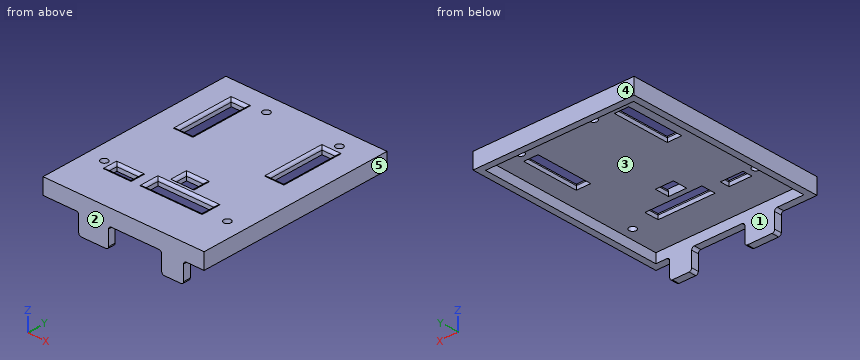
from build123d import *

# Parameters (mm, degrees)
SKETCH018_W   = 61.65
SKETCH018_H   = 75.98
SKETCH018_R   = 1.375
SKETCH018_W_2 = 21.82
SKETCH018_H_2 = 5.5
SKETCH018_W_3 = 8.7
SKETCH018_H_3 = 3.63
SKETCH018_W_4 = 6.9
SKETCH018_W_5 = 5.5
SKETCH018_H_4 = 21.975
SKETCH018_H_5 = 21.865
PAD011_DEPTH  = 2.5
SKETCH019_W   = 61.65
SKETCH019_H   = 75.98
SKETCH019_W_2 = 56.65
SKETCH019_H_2 = 70.73
PAD012_DEPTH  = 3.6
SKETCH020_W   = 11.43
SKETCH020_H   = 2.75
SKETCH020_W_2 = 8.39
PAD013_DEPTH  = 11.35
FILLET005_R   = 1


with BuildPart() as part:
    # Sketch018 → Pad011 (new body)
    with BuildSketch(Plane.XY):
        with Locations((0, -30.5)):
            Rectangle(SKETCH018_W, SKETCH018_H)
        with Locations((-8.89, 0.5)):
            Circle(SKETCH018_R, mode=Mode.SUBTRACT)
        with Locations((19.05, 0.5)):
            Circle(SKETCH018_R, mode=Mode.SUBTRACT)
        with Locations((-24.13, -50.3)):
            Circle(SKETCH018_R, mode=Mode.SUBTRACT)
        with Locations((24.13, -51.57)):
            Circle(SKETCH018_R, mode=Mode.SUBTRACT)
        with Locations((4.49, -49.92)):
            Rectangle(SKETCH018_W_2, SKETCH018_H_2, mode=Mode.SUBTRACT)
        with Locations((-16.12, -50.855)):
            Rectangle(SKETCH018_W_3, SKETCH018_H_3, mode=Mode.SUBTRACT)
        with Locations((1.03, -42.42)):
            Rectangle(SKETCH018_W_4, SKETCH018_H_2, mode=Mode.SUBTRACT)
        with Locations((-18.4, -11.7825)):
            Rectangle(SKETCH018_W_5, SKETCH018_H_4, mode=Mode.SUBTRACT)
        with Locations((18.475, -14.0775)):
            Rectangle(SKETCH018_W_5, SKETCH018_H_5, mode=Mode.SUBTRACT)
    extrude(amount=PAD011_DEPTH)

    # Sketch019 → Pad012 (join)
    with BuildSketch(Plane.XY):
        with Locations((0, -30.5)):
            Rectangle(SKETCH019_W, SKETCH019_H)
        with Locations((0, -30.375)):
            Rectangle(SKETCH019_W_2, SKETCH019_H_2, mode=Mode.SUBTRACT)
    extrude(amount=-PAD012_DEPTH)

    # Sketch020 → Pad013 (join)
    with BuildSketch(Plane.XY):
        with Locations((-11.43, -67.115)):
            Rectangle(SKETCH020_W, SKETCH020_H)
        with Locations((18.8, -67.115)):
            Rectangle(SKETCH020_W_2, SKETCH020_H)
    extrude(amount=-PAD013_DEPTH)

    # Fillet005
    fillet005_edges = [part.edges().sort_by_distance(p)[0] for p in [
        (-20.47, -50.855, 2.5),
        (-16.12, -49.04, 2.5),
        (-16.12, -52.67, 2.5),
        (-11.77, -50.855, 2.5),
        (-6.42, -49.92, 2.5),
        (4.49, -47.17, 2.5),
        (4.49, -52.67, 2.5),
        (15.4, -49.92, 2.5),
        (-2.42, -42.42, 2.5),
        (1.03, -39.67, 2.5),
        (4.48, -42.42, 2.5),
        (18.475, -3.145, 2.5),
        (21.225, -14.0775, 2.5),
        (15.725, -14.0775, 2.5),
        (18.475, -25.01, 2.5),
        (-18.4, -0.795, 2.5),
        (-15.65, -11.7825, 2.5),
        (-21.15, -11.7825, 2.5),
        (-18.4, -22.77, 2.5),
        (-17.145, -67.115, -3.6),
        (-17.145, -67.115, -11.35),
        (-5.715, -67.115, -11.35),
        (14.605, -67.115, -3.6),
        (14.605, -67.115, -11.35),
        (22.995, -67.115, -11.35),
        (-5.715, -67.115, -3.6),
        (22.995, -67.115, -3.6),
    ]]
    fillet(fillet005_edges, radius=FILLET005_R)


solid = part.part
The model under review builds one solid part; all positions refer to its coordinate system, in mm. Face numbers are marked on the shaded views. A direction names the side the tool comes from. Round coordinates to 2 decimals unless told otherwise and drop trailing zeros. Write each loop counter-clockwise with the first axis right and the second up, starting at its lowest first coordinate (ties: lowest second). Pieces come first, ordered by that corner, then holes. Notation, with made-up numbers: (-14.5, 49.25) - (11.5, 49.25) arc R15 ccw to (11.5, 64.25) - close; hole circle Ø7 at (-38.5, 26). An arc over 180 degrees is marked (long way). One line per item, written item: value. Start each with the question number.
1. Consider section C-C on z = -8.5. Write out the cut boundary in (x, y) (3 decimals).
2. Machinability: for the marked faces 1 and 2, which of the approach directions +Z, -Z, +X, -X, +Y, -Y give a long, thin tool a straight path to every point of the face, cutting with its end or side? Answer none if there is none.
3. The part is to be moulded in two halves that separate along X. For the marked faces 3, 4 and 5, say which applies: released by +X, released by -X, zero draft, split by the parting line, or undercut.
4. Consider section B-B on z = -1.75. Write out the cut boundary in (x, y) (3 decimals), and give its area (3 significant figures).
5. Consider section A-A on x = 19.05. Write out the cut boundary in (y, z) (3 decimals).
6. Clearance check with flat-ended pins moving along their axes: P1, Ø2.5, axis at x = 24.13, y = -51.57, coming from the +Z side; P2, Ø2, axis at y = -67.5, z = -7, coming from the +X side (3 decimals); P3, Ø2, axis at y = -67, z = -6.5, coming from the -X side (3 decimals); P4, Ø2, axis at x = -23.5, y = -60.5, coming from the -Z side. State where each tip first meets the part, or that it passes through.
7. Consider section D-D on x = -24.13. Write out the cut boundary in (y, z) (3 decimals).
8. To check wall thickness, follow L1, parallel to Y at x = -8.89, z = 0.9 (3 decimals); L2, parallel to Y at x = 18.5, z = -1.5; L3, parallel to X at y = -30, z = -1.5 (3 decimals). State the ranges of each line that lie inside material, in increasing order. Write a range as from..to.
Checks:
1. outline: (-17.145, -68.49) - (-5.715, -68.49) - (-5.715, -65.74) - (-17.145, -65.74) - close; (14.605, -68.49) - (22.995, -68.49) - (22.995, -65.74) - (14.605, -65.74) - close
2. face 1: -Z
2. face 2: +Z, -Z, +X, -X, -Y
3. face 3: undercut
3. face 4: zero draft
3. face 5: released by +X
4. outline: (-30.825, -68.49) - (30.825, -68.49) - (30.825, 7.49) - (-30.825, 7.49) - close; hole (-28.325, -65.74) - (28.325, -65.74) - (28.325, 4.99) - (-28.325, 4.99) - close
4. area: 677 mm^2
5. outline: (-68.49, -11.35) - (-65.74, -11.35) - (-65.74, 0) - (-25.01, 0) - (-25.01, 1.5) arc R1 ccw to (-26.01, 2.5) - (-68.49, 2.5) - close; (-3.145, 0) - (-0.875, 0) - (-0.875, 2.5) - (-2.145, 2.5) arc R1 ccw to (-3.145, 1.5) - close; (1.875, 0) - (4.99, 0) - (4.99, -3.6) - (7.49, -3.6) - (7.49, 2.5) - (1.875, 2.5) - close
6. P1: passes through
6. P2: stops at x = 22.995
6. P3: stops at x = -17.145
6. P4: stops at z = 0
7. outline: (-68.49, -3.6) - (-65.74, -3.6) - (-65.74, 0) - (-51.675, 0) - (-51.675, 2.5) - (-68.49, 2.5) - close; (-48.925, 0) - (4.99, 0) - (4.99, -3.6) - (7.49, -3.6) - (7.49, 2.5) - (-48.925, 2.5) - close
8. L1: y = -68.49..-0.875, 1.875..7.49
8. L2: y = -68.49..-65.74, 4.99..7.49
8. L3: x = -30.825..-28.325, 28.325..30.825
